Autodesk Inventor part; units mm, degrees
ref_plane "YZ Plane" through (0, 0, 0) normal (1, 0, 0) x (0, 1, 0)
ref_plane "XZ Plane" through (0, 0, 0) normal (0, 1, 0) x (-1, 0, 0)
ref_plane "XY Plane" through (0, 0, 0) normal (0, 0, 1) x (1, 0, 0)
sketch "Sketch1" plane through (0, 0, 0) normal (0, 1, 0) x (-1, 0, 0)
  circle A0 centre (-31.75, 0) radius 11.0744
  circle A1 centre (24.765, 0) radius 9.652
  line L0 (-16.51, -6.35) -> (11.9662, -6.35)
  circle A2 centre (24.765, 0) radius 14.2875
  circle A3 centre (-31.75, 0) radius 16.51
  line L1 (-16.51, 6.35) -> (11.9662, 6.35)
  point P0 (0, 0)
  dimension "d15" = 22.1488
  dimension "d17" = 12.7
  dimension "d18" = 33.02
  dimension "d19" = 19.304
  dimension "d20" = 28.575
  dimension "d21" = 56.515
extrude "Extrusion2" add sketch "Sketch1" along normal blind 7.62 contours A0 | A1 | A3 L1 A2 L0 | A3 | A2
fillet "Fillet3" radius 25.4 4 edges at (-11.9662, 3.81, 6.35) (-11.9662, 3.81, -6.35) (16.51, 3.81, -6.35) (16.51, 3.81, 6.35)
draft "FaceDraft2" angle 3 pull direction (0, 1, 0) faces at (41.7415, 5.08, -13.1435) (14.1702, 2.54, 8.307) (8.391, 2.54, -6.6666) (0.8295, 2.54, 6.35) (2.6114, 2.54, -6.35) (-2.7671, 2.54, 6.4149) (-4.5723, 2.54, -6.6093) (-18.1739, 5.08, 12.6764) fixed edges at (48.26, 0, 0) (13.2365, 0, 7.9391) (13.2365, 0, -7.9391) (1.7204, 0, 6.35) (1.7204, 0, -6.35) (-8.9847, 0, 7.6534) (-8.9847, 0, -7.6534) (-39.0525, 0, 0)
properties part number "Connecting Rod Cast Image"
Build history of the part. All positions in model axes, mm. Coordinates: 2 decimals unless noted, no trailing zeros. Answer in a Markdown table with one row per item. Add a question column.
Q1. Drop flat-ended pins along their axis: pin 1 (3 mm diameter, centred on x = 4, z = 4.5, fed in from -Y); pin 2 (3 mm diameter, centred on x = 14, y = 4.5, fed in from +Z). Give the stop position or say it passes through.
Q2. Mould opens along X. For faces 1 (the face through (1.758, 3.757, 6.153)), 2 (the face through (5, 0, 0)), 3 (the face through (1.758, 3.757, -6.153)) say: +X half, -X half, draft (parallel to the pull), parting line (faces both ways), or undercut.
Q3. Wall check: line 1 along Z through (x, y) = (34.5, 3); line 2 along X through (y, z) = (2.75, 11); line 3 along X through (y, z) = (7, 11). Give the ranges that are in metal, low to high. Write a range as [from, to].
Answers follow:
| question | item | result |
|---|---|---|
| 1 | pin 1 | y = 0 |
| 1 | pin 2 | z = 8.65 |
| 2 | face 1 | undercut |
| 2 | face 2 | draft |
| 2 | face 3 | undercut |
| 3 | line 1 | [-16.12, 16.12] |
| 3 | line 2 | [-33.66, -15.85], [19.29, 43.87] |
| 3 | line 3 | [-33.3, -16.23], [19.67, 43.57] |
